The listing builds one solid part. Answer for the finished solid, in the listing's coordinates (mm). A direction names the side the tool comes from. Coordinates: 2 decimals unless noted, no trailing zeros. Order: outer loops, then holes, each group sorted by start corner. A loop starts at its lowest first (then second) coordinate and runs counter-clockwise, first axis right, second up. Notation, with made-up numbers: (-39.75, -20) -> (18.25, -20) arc R20 cw to (18.25, 13) -> close; hole circle Ø4 at (18, 10.25). An arc over 180 degrees is marked (long way). Answer in a Markdown table with one row per item.
```python
from build123d import *

# Parameters (mm, degrees)
SKETCH1_R           = 1.6
BOSS_EXTRUDE1_DEPTH = 2
BOSS_EXTRUDE3_DEPTH = 10
CUT_EXTRUDE2_DEPTH  = 26.38700455
CUT_EXTRUDE3_DEPTH  = 8
CHAMFER1_SIZE       = 1
FILLET4_R           = 1
CHAMFER2_SIZE       = 1


with BuildPart() as part:
    # Sketch1 → Boss-Extrude1 (new body)
    with BuildSketch(Plane.XY):
        with BuildLine():
            Line((-12.5, -16.5), (12.5, -16.5))
            ThreePointArc((12.5, -16.5), (15.328427125, -15.328427125), (16.5, -12.5))
            Line((16.5, -12.5), (16.5, 12.5))
            ThreePointArc((16.5, 12.5), (15.328427125, 15.328427125), (12.5, 16.5))
            Line((12.5, 16.5), (-12.5, 16.5))
            ThreePointArc((-12.5, 16.5), (-15.328427125, 15.328427125), (-16.5, 12.5))
            Line((-16.5, 12.5), (-16.5, -12.5))
            ThreePointArc((-16.5, -12.5), (-15.328427125, -15.328427125), (-12.5, -16.5))
        make_face()
        with Locations((-12.5, -12.5)):
            Circle(SKETCH1_R, mode=Mode.SUBTRACT)
        with Locations((12.5, -12.5)):
            Circle(SKETCH1_R, mode=Mode.SUBTRACT)
        with Locations((12.5, 12.5)):
            Circle(SKETCH1_R, mode=Mode.SUBTRACT)
        with Locations((-12.5, 12.5)):
            Circle(SKETCH1_R, mode=Mode.SUBTRACT)
    extrude(amount=BOSS_EXTRUDE1_DEPTH)

    # Sketch3 → Boss-Extrude3 (add)
    with BuildSketch(Plane.XY):
        with BuildLine():
            ThreePointArc((6, -12.649110641), (0, 14), (-6, -12.649110641))
            Line((-6, -12.649110641), (-6, -16.5))
            Line((-6, -16.5), (6, -16.5))
            Line((6, -16.5), (6, -12.649110641))
        make_face()
    extrude(amount=BOSS_EXTRUDE3_DEPTH)

    # Sketch3_3 → Cut-Extrude2 (cut, through all)
    with BuildSketch(Plane.XY):
        with BuildLine():
            Line((-11.169539803, -1.25), (-9.669539803, -1.25))
            ThreePointArc((-9.669539803, -1.25), (-7.15797616, -6.620111577), (-2, -9.542667342))
            Line((-2, -9.542667342), (-2, -12.542667342))
            Line((-2, -12.542667342), (2, -12.542667342))
            Line((2, -12.542667342), (2, -9.542667342))
            ThreePointArc((2, -9.542667342), (9.75, 0), (2, 9.542667342))
            Line((2, 9.542667342), (2, 12.542667342))
            Line((2, 12.542667342), (-2, 12.542667342))
            Line((-2, 12.542667342), (-2, 9.542667342))
            ThreePointArc((-2, 9.542667342), (-7.15797616, 6.620111577), (-9.669539803, 1.25))
            Line((-9.669539803, 1.25), (-11.169539803, 1.25))
            Line((-11.169539803, 1.25), (-11.169539803, -1.25))
        make_face()
    extrude(amount=CUT_EXTRUDE2_DEPTH, mode=Mode.SUBTRACT)

    # Sketch3_4 → Cut-Extrude3 (cut)
    with BuildSketch(Plane.XY):
        with BuildLine():
            ThreePointArc((-2, -9.542667342), (-3.017604429, -9.271276261), (-4, -8.891709622))
            Line((-4, -8.891709622), (-4, -16.5))
            Line((-4, -16.5), (4, -16.5))
            Line((4, -16.5), (4, -8.891709622))
            ThreePointArc((4, -8.891709622), (3.017604429, -9.271276261), (2, -9.542667342))
            Line((2, -9.542667342), (2, -12.542667342))
            Line((2, -12.542667342), (-2, -12.542667342))
            Line((-2, -12.542667342), (-2, -9.542667342))
        make_face()
    extrude(amount=CUT_EXTRUDE3_DEPTH, mode=Mode.SUBTRACT)

    # Chamfer1
    chamfer1_edges = [part.edges().sort_by_distance(p)[0] for p in [
        (-15.328427125, -15.328427125, 2),
        (-9.25, -16.5, 2),
        (15.328427125, -15.328427125, 2),
        (16.5, 0, 2),
        (15.328427125, 15.328427125, 2),
        (0, 16.5, 2),
        (9.25, -16.5, 2),
        (-15.328427125, 15.328427125, 2),
        (-16.5, 0, 2),
    ]]
    chamfer(chamfer1_edges, length=CHAMFER1_SIZE)

    # Fillet4
    fillet4_edges = [part.edges().sort_by_distance(p)[0] for p in [
        (0, 14, 2),
        (6, -14.57455532, 10),
        (0, 14, 10),
        (-6, -14.57455532, 10),
    ]]
    fillet(fillet4_edges, radius=FILLET4_R)

    # Chamfer2
    chamfer2_edges = [part.edges().sort_by_distance(p)[0] for p in [
        (-6, -16.5, 5),
        (6, -16.5, 5),
        (-5.707106781, -16.5, 9.707106781),
        (5.707106781, -16.5, 9.707106781),
        (0, -16.5, 10),
    ]]
    chamfer(chamfer2_edges, length=CHAMFER2_SIZE)


solid = part.part
```
(1) For a pull along X with two mould halves and no side action, classify faces 1 (the conical face through (5.362, -15.993, 9.355)), 2 (the flat face through (-6, -14, 5)), 3 (the cylindrical face through (-8.045, -5.509, 4.93)) as released by +X, released by -X, zero draft, split by the parting line, or undercut.
Check values:
| item | result |
|---|---|
| face 1 | released by +X |
| face 2 | released by -X |
| face 3 | undercut |
(2) A cutting plane is placed at A-A, the plane x = 0. Determine the outline of the cut face in (y, z).
Check values:
| item | result |
|---|---|
| outline | (-16.5, 8) -> (-12.54, 8) -> (-12.54, 10) -> (-15.5, 10) -> (-16.5, 9) -> close; (12.54, 0) -> (16.5, 0) -> (16.5, 1) -> (15.5, 2) -> (15, 2) arc R1 cw to (14, 3) -> (14, 9) arc R1 ccw to (13, 10) -> (12.54, 10) -> close |
(3) A cutting plane is placed at D-D, the plane y = 13.5. Count the separate pieces of the cut face and the enclosed holes in it, then the cut area to 3 significant figures.
Check values:
| item | result |
|---|---|
| separate pieces | 3 |
| enclosed holes | 0 |
| area | 113 mm² |
(4) Which of the six approach directions +Z, -Z, +X, -X, +Y, -Y give full straight-line access (tool end or side, diameter ignored) to faces 4 (the flat face through (-10, -1.25, 5)), 5 (the conical face through (-14.797, 14.848, 1.715)), 6 (the flat face through (4, -13, 4))?
Check values:
| item | result |
|---|---|
| face 4 | +Z, -Z |
| face 5 | +Z, -X, +Y |
| face 6 | -Z, -Y |
(5) Flat-ended cylindrical pins translate along their axes: pin 1 (1.6 mm diameter, centred on y = -10.5, z = 9, fed in from +X); pin 2 (6 mm diameter, centred on y = 1.5, z = 5.5, fed in from +X); pin 3 (5 mm diameter, centred on x = 12.5, y = -12.5, fed in from -Z); pin 4 (1.5 mm diameter, centred on y = 11.5, z = 6.5, fed in from +X). Find the tip coordinate at first contact, or state that the pin passes through.
Check values:
| item | result |
|---|---|
| pin 1 | x = 10.1 |
| pin 2 | x = 14.08 |
| pin 3 | z = 0 |
| pin 4 | x = 8.97 |
(6) Find the intervals of material crossed by line 1 along Y through (x, z) = (12.5, 0.55); line 2 along X through (y, z) = (-14, 7); line 3 along Y through (x, z) = (5.5, 4.5), in increasing order. Write a range as from..to.
Check values:
| item | result |
|---|---|
| line 1 | -16.5..-14.1, -10.9..10.9, 14.1..16.5 |
| line 2 | -6..-4, 4..6 |
| line 3 | -16..-8.05, 8.05..12.87 |
(7) A cutting plane is placed at B-B, the plane z = 8.5. Determine the outline of the cut face in (x, y), then the cut area to 3 significant figures.
Check values:
| item | result |
|---|---|
| outline | (-6, -15.5) -> (-5, -16.5) -> (5, -16.5) -> (6, -15.5) -> (6, -12.65) arc R14 ccw (long way) to (-6, -12.65) -> close; hole (-11.17, -1.25) -> (-9.67, -1.25) arc R9.75 ccw to (-2, -9.54) -> (-2, -12.54) -> (2, -12.54) -> (2, -9.54) arc R9.75 ccw to (2, 9.54) -> (2, 12.54) -> (-2, 12.54) -> (-2, 9.54) arc R9.75 ccw to (-9.67, 1.25) -> (-11.17, 1.25) -> close |
| area | 325 mm² |
(8) A cutting plane is placed at C-C, the plane z = 6.25. Determine the outline of the cut face in (x, y).
Check values:
| item | result |
|---|---|
| outline | (-11.17, -1.25) -> (-11.17, 1.25) -> (-9.67, 1.25) arc R9.75 cw to (-2, 9.54) -> (-2, 12.54) -> (2, 12.54) -> (2, 9.54) arc R9.75 cw to (4, -8.89) -> (4, -16.5) -> (5, -16.5) -> (6, -15.5) -> (6, -12.65) arc R14 ccw (long way) to (-6, -12.65) -> (-6, -15.5) -> (-5, -16.5) -> (-4, -16.5) -> (-4, -8.89) arc R9.75 cw to (-9.67, -1.25) -> close |
